Geometry check sheet. Reference: the model listing, model coordinates, mm. A direction names the side the tool comes from. Give positions to 0.01 mm unless a question says otherwise; leave off trailing zeros. Loops run counter-clockwise (first coordinate to the right, second up) from the corner with the lowest first, then second, coordinate; pieces in that order, holes last.
1. Tool access check on faces 1 (the flat face through (-20, 20, 7)), 2 (the flat face through (6, -17, 8)). Record the directions out of +Z, -Z, +X, -X, +Y, -Y that give a thin tool (end or side, any length) a straight path to the whole face; none if there is none.
2. Cross-section at A-A, the plane x = -32. Record the cut outline in (y, z).
3. Material ranges on L1, parallel to X at y = 13, z = 5.25; L2, parallel to X at y = 15, z = 13.75; L3, parallel to Y at x = 0.5, z = 13, recorded low to high.
4. Release check for a two-part mould opening along X. For faces 3 (the flat face through (12, -20, 7)), 4 (the cylindrical face through (-32, 18, 8)) record: +X half, -X half, draft (parallel to the pull), parting line (faces both ways), or undercut.
from build123d import *

# Parameters (mm, degrees)
SKETCH1_W                                = 200
SKETCH1_H                                = 40
RECTANGULAR_BAR_40_W_X_200_L_X_15D_DEPTH = 15
NOTCH_CUT_OUT_DEPTH                      = 15
CUT_EXTRUDE1_DEPTH                       = 16


with BuildPart() as part:
    # Sketch1 → Rectangular Bar (40 W x 200 L x 15D) (new body)
    with BuildSketch(Plane.XY):
        Rectangle(SKETCH1_W, SKETCH1_H)
    extrude(amount=RECTANGULAR_BAR_40_W_X_200_L_X_15D_DEPTH)

    # Notch → Notch cut out (cut)
    with BuildSketch(Plane.XY.offset(15)):
        with BuildLine():
            Line((2, 20), (2, 12))
            ThreePointArc((2, 12), (0, 10), (-2, 12))
            Line((-2, 12), (-2, 20))
            Line((-2, 20), (2, 20))
        make_face()
        with BuildLine():
            Line((-2, -20), (-2, -12))
            ThreePointArc((-2, -12), (0, -10), (2, -12))
            Line((2, -12), (2, -20))
            Line((2, -20), (-2, -20))
        make_face()
    extrude(amount=-NOTCH_CUT_OUT_DEPTH, mode=Mode.SUBTRACT)

    # Sketch2 → Cut-Extrude1 (cut, through all)
    with BuildSketch(Plane.XY.offset(15)):
        with BuildLine():
            Line((6, 20), (6, 14))
            ThreePointArc((6, 14), (8, 12), (10, 14))
            Line((10, 14), (10, 20))
            Line((10, 20), (6, 20))
        make_face()
        with BuildLine():
            Line((14, 20), (14, 16))
            ThreePointArc((14, 16), (16, 14), (18, 16))
            Line((18, 16), (18, 20))
            Line((18, 20), (14, 20))
        make_face()
        with BuildLine():
            Line((22, 20), (22, 18))
            ThreePointArc((22, 18), (24, 16), (26, 18))
            Line((26, 18), (26, 20))
            Line((26, 20), (22, 20))
        make_face()
        with BuildLine():
            Line((30, 20), (34, 20))
            ThreePointArc((34, 20), (32, 18), (30, 20))
        make_face()
        with BuildLine():
            Line((-30, 20), (-34, 20))
            ThreePointArc((-34, 20), (-32, 18), (-30, 20))
        make_face()
        with BuildLine():
            Line((-22, 20), (-26, 20))
            Line((-26, 20), (-26, 18))
            ThreePointArc((-26, 18), (-24, 16), (-22, 18))
            Line((-22, 18), (-22, 20))
        make_face()
        with BuildLine():
            Line((-18, 20), (-18, 16))
            ThreePointArc((-18, 16), (-16, 14), (-14, 16))
            Line((-14, 16), (-14, 20))
            Line((-14, 20), (-18, 20))
        make_face()
        with BuildLine():
            Line((-10, 20), (-10, 14))
            ThreePointArc((-10, 14), (-8, 12), (-6, 14))
            Line((-6, 14), (-6, 20))
            Line((-6, 20), (-10, 20))
        make_face()
        with BuildLine():
            Line((30, -20), (34, -20))
            ThreePointArc((34, -20), (32, -18), (30, -20))
        make_face()
        with BuildLine():
            Line((26, -20), (26, -18))
            ThreePointArc((26, -18), (24, -16), (22, -18))
            Line((22, -18), (22, -20))
            Line((22, -20), (26, -20))
        make_face()
        with BuildLine():
            Line((18, -20), (18, -16))
            ThreePointArc((18, -16), (16, -14), (14, -16))
            Line((14, -16), (14, -20))
            Line((14, -20), (18, -20))
        make_face()
        with BuildLine():
            Line((10, -20), (10, -14))
            ThreePointArc((10, -14), (8, -12), (6, -14))
            Line((6, -14), (6, -20))
            Line((6, -20), (10, -20))
        make_face()
        with BuildLine():
            Line((-6, -20), (-6, -14))
            ThreePointArc((-6, -14), (-8, -12), (-10, -14))
            Line((-10, -14), (-10, -20))
            Line((-10, -20), (-6, -20))
        make_face()
        with BuildLine():
            Line((-14, -20), (-14, -16))
            ThreePointArc((-14, -16), (-16, -14), (-18, -16))
            Line((-18, -16), (-18, -20))
            Line((-18, -20), (-14, -20))
        make_face()
        with BuildLine():
            Line((-30, -20), (-34, -20))
            ThreePointArc((-34, -20), (-32, -18), (-30, -20))
        make_face()
        with BuildLine():
            Line((-22, -20), (-22, -18))
            ThreePointArc((-22, -18), (-24, -16), (-26, -18))
            Line((-26, -18), (-26, -20))
            Line((-26, -20), (-22, -20))
        make_face()
    extrude(amount=-CUT_EXTRUDE1_DEPTH, mode=Mode.SUBTRACT)


solid = part.part
Result:
1. face 1: +Z, -Z, +X, -X, +Y
1. face 2: +Z, -Z, -Y
2. outline: (-18, 0) - (18, 0) - (18, 15) - (-18, 15) - close
3. L1: x = -100 to -9.73, -6.27 to -2, 2 to 6.27, 9.73 to 100
3. L2: x = -100 to -17.73, -14.27 to -10, -6 to -2, 2 to 6, 10 to 14.27, 17.73 to 100
3. L3: y = -10.06 to 10.06
4. face 3: draft
4. face 4: undercut
